Verification items for the finished model (mm, model axes). Face numbers are marked on the shaded views. A direction names the side the tool comes from. Round coordinates to 2 decimals unless told otherwise and drop trailing zeros. Loops run counter-clockwise (first coordinate to the right, second up) from the corner with the lowest first, then second, coordinate; pieces in that order, holes last. Notation, with made-up numbers: M 77,85 L 105,85 A16 ccw 105,90 Z; hole C 78,-39.5 d3. An arc over 180 degrees is marked long. Write item = value, one per line. Start each with the question number.
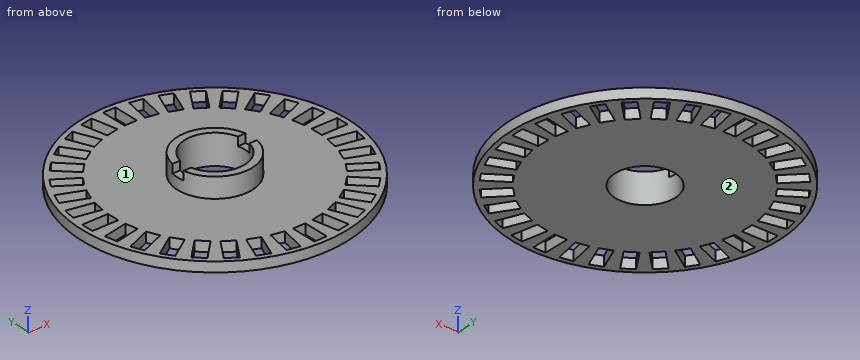
from build123d import *

# Parameters (mm, degrees)
SKETCH_R        = 26.7
PAD_DEPTH       = 2
SKETCH001_W     = 5.2
SKETCH001_H     = 2.5
SKETCH001_W_2   = 2.5
SKETCH001_H_2   = 5.2
POCKET_DEPTH    = 2.001
SKETCH002_R     = 7.5
PAD001_DEPTH    = 4
SKETCH003_R     = 6
POCKET001_DEPTH = 6.001
SKETCH004_W     = 18.225545
SKETCH004_H     = 2.75
POCKET002_DEPTH = 1.75


with BuildPart() as part:
    # Sketch → Pad (new body)
    with BuildSketch(Plane.XY):
        Circle(SKETCH_R)
    extrude(amount=PAD_DEPTH)

    # Sketch001 → Pocket (cut, through all)
    with BuildSketch(Plane.XY.offset(2)):
        with Locations((-23.1, 0)):
            Rectangle(SKETCH001_W, SKETCH001_H)
        with Locations((23.1, 0)):
            Rectangle(SKETCH001_W, SKETCH001_H)
        with Locations((0, 23.1)):
            Rectangle(SKETCH001_W_2, SKETCH001_H_2)
        with Locations((0, -23.1)):
            Rectangle(SKETCH001_W_2, SKETCH001_H_2)
        Polygon((-19.029555, 17.261788), (-17.261788, 19.029555), (-13.584833, 15.3526), (-15.3526, 13.584833), align=None)
        Polygon((17.261788, 19.029555), (19.029555, 17.261788), (15.3526, 13.584833), (13.584833, 15.3526), align=None)
        Polygon((17.261788, -19.029555), (19.029555, -17.261788), (15.3526, -13.584833), (13.584833, -15.3526), align=None)
        Polygon((-17.261788, -19.029555), (-19.029555, -17.261788), (-15.3526, -13.584833), (-13.584833, -15.3526), align=None)
        Polygon((8.680115, 24.222058), (6.690161, 19.417885), (8.99986, 18.461176), (10.989814, 23.26535), align=None)
        Polygon((18.461176, 8.99986), (19.417885, 6.690161), (24.037282, 8.603578), (23.080574, 10.913277), align=None)
        Polygon((-23.26535, 10.989814), (-24.222058, 8.680115), (-19.417885, 6.690161), (-18.461176, 8.99986), align=None)
        Polygon((-24.222058, -8.680115), (-23.26535, -10.989814), (-18.461176, -8.99986), (-19.417885, -6.690161), align=None)
        Polygon((-10.989814, -23.26535), (-8.680115, -24.222058), (-6.690161, -19.417885), (-8.99986, -18.461176), align=None)
        Polygon((6.690161, -19.417885), (8.680115, -24.222058), (10.989814, -23.26535), (8.99986, -18.461176), align=None)
        Polygon((19.417885, -6.690161), (18.461176, -8.99986), (23.26535, -10.989814), (24.222058, -8.680115), align=None)
        Polygon((-10.989814, 23.26535), (-8.680115, 24.222058), (-6.690161, 19.417885), (-8.99986, 18.461176), align=None)
        Polygon((19.862235, 5.225333), (20.349961, 2.77337), (25.253888, 3.748822), (24.766162, 6.200785), align=None)
        Polygon((-25.253888, -3.748822), (-24.766162, -6.200785), (-19.862235, -5.225333), (-20.349961, -2.77337), align=None)
        Polygon((-24.962319, 6.239803), (-25.450045, 3.78784), (-20.349961, 2.77337), (-19.862235, 5.225333), align=None)
        Polygon((-20.778522, 15.161523), (-21.959016, 13.394787), (-17.635375, 10.505822), (-16.45488, 12.272558), align=None)
        Polygon((-15.317492, 20.674306), (-13.238818, 22.063232), (-10.349853, 17.73959), (-12.428527, 16.350664), align=None)
        Polygon((-6.241651, 24.971611), (-3.789688, 25.459337), (-2.775218, 20.359254), (-5.227182, 19.871528), align=None)
        Polygon((3.78784, 25.450045), (2.77337, 20.349961), (5.225333, 19.862235), (6.239803, 24.962319), align=None)
        Polygon((13.238818, 22.063232), (10.349853, 17.73959), (12.428527, 16.350664), (15.317492, 20.674306), align=None)
        Polygon((16.350664, 12.428527), (17.73959, 10.349853), (22.063232, 13.238818), (20.674306, 15.317492), align=None)
        Polygon((20.349961, -2.77337), (19.862235, -5.225333), (24.962319, -6.239803), (25.450045, -3.78784), align=None)
        Polygon((17.635375, -10.505822), (16.45488, -12.272558), (20.778522, -15.161523), (21.959016, -13.394787), align=None)
        Polygon((10.349853, -17.73959), (12.428527, -16.350664), (15.317492, -20.674306), (13.238818, -22.063232), align=None)
        Polygon((2.775218, -20.359254), (5.227182, -19.871528), (6.241651, -24.971611), (3.789688, -25.459337), align=None)
        Polygon((-2.77337, -20.349961), (-3.78784, -25.450045), (-6.239803, -24.962319), (-5.225333, -19.862235), align=None)
        Polygon((-15.317492, -20.674306), (-13.238818, -22.063232), (-10.349853, -17.73959), (-12.428527, -16.350664), align=None)
        Polygon((-22.063232, -13.238818), (-20.674306, -15.317492), (-16.350664, -12.428527), (-17.73959, -10.349853), align=None)
    extrude(amount=-POCKET_DEPTH, mode=Mode.SUBTRACT)

    # Sketch002 → Pad001 (new body)
    with BuildSketch(Plane.XY.offset(2)):
        Circle(SKETCH002_R)
    extrude(amount=PAD001_DEPTH)

    # Sketch003 → Pocket001 (cut, through all)
    with BuildSketch(Plane.XY.offset(6)):
        Circle(SKETCH003_R)
    extrude(amount=-POCKET001_DEPTH, mode=Mode.SUBTRACT)

    # Sketch004 → Pocket002 (cut)
    with BuildSketch(Plane.XY.offset(6)):
        with Locations((0.188303, 0.078437)):
            Rectangle(SKETCH004_W, SKETCH004_H)
    extrude(amount=-POCKET002_DEPTH, mode=Mode.SUBTRACT)


solid = part.part
1. Gauge pin test, flat ends, axial feed: P1, Ø2, axis at y = 22.5, z = 1, coming from the -X side; P2, Ø5, axis at x = 15, y = 16.5, coming from the +Z side; P3, Ø2, axis at y = -22, z = 1.5, coming from the -X side; P4, Ø11, axis at x = 0, y = 0, coming from the -Z side. Record the tip position at first contact, or that the pin passes through.
2. Thickness scan on line 1 (Y direction, x = 0, z = 1.6); line 2 (Y direction, x = 0, z = 2.8); line 3 (Y direction, x = 14, z = 0.85). Record the ranges inside material, lowest first.
3. Section check C-C, the plane z = 5.25. Enter the section's corners in (x, y), and give its area (3 significant figures).
4. Section check B-B, the plane x = 0. Enter the section's corners in (y, z), and give its area (3 significant figures).
5. Section check D-D, the plane y = -14.5. Enter the section's corners in (x, z).
6. Section check A-A, the plane y = 0. Enter the section's corners in (x, z), and give its area (4 significant figures).
7. Tool access check on the marked faces 1 and 2. Record the directions out of +Z, -Z, +X, -X, +Y, -Y that give a thin tool (end or side, any length) a straight path to the whole face; none if there is none.
Computed values:
q1.P1 = -15.83
q1.P2 = 2
q1.P3 = -16.49
q1.P4 = through
q2.line_1 = -26.7 to -25.7, -20.5 to -6, 6 to 20.5, 25.7 to 26.7
q2.line_2 = -7.5 to -6, 6 to 7.5
q2.line_3 = -22.74 to -21.55, -18.7 to -15.77, -14.94 to 14.94, 15.77 to 18.7, 21.55 to 22.74
q3.outline = M -7.39,-1.3 A7.5 ccw 7.39,-1.3 L 5.86,-1.3 A6 cw -5.86,-1.3 Z; M -7.36,1.45 L -5.82,1.45 A6 cw 5.82,1.45 L 7.36,1.45 A7.5 ccw Z
q3.area = 55.3 mm2
q4.outline = M -26.7,0 L -25.7,0 L -25.7,2 L -26.7,2 Z; M -20.5,0 L -6,0 L -6,6 L -7.5,6 L -7.5,2 L -20.5,2 Z; M 6,0 L 20.5,0 L 20.5,2 L 7.5,2 L 7.5,6 L 6,6 Z; M 25.7,0 L 26.7,0 L 26.7,2 L 25.7,2 Z
q4.area = 74.0 mm2
q5.outline = M -22.42,0 L -21.22,0 L -21.22,2 L -22.42,2 Z; M -19.45,0 L -16.27,0 L -16.27,2 L -19.45,2 Z; M -14.44,0 L 14.44,0 L 14.44,2 L -14.44,2 Z; M 16.27,0 L 19.79,0 L 19.79,2 L 16.27,2 Z; M 21.22,0 L 22.42,0 L 22.42,2 L 21.22,2 Z
q6.outline = M -26.7,0 L -25.7,0 L -25.7,2 L -26.7,2 Z; M -20.5,0 L -6,0 L -6,4.25 L -7.5,4.25 L -7.5,2 L -20.5,2 Z; M 6,0 L 20.5,0 L 20.5,2 L 7.5,2 L 7.5,4.25 L 6,4.25 Z; M 25.7,0 L 26.7,0 L 26.7,2 L 25.7,2 Z
q6.area = 68.75 mm2
q7.face_1 = +Z
q7.face_2 = -Z, +X, -X, +Y, -Y
